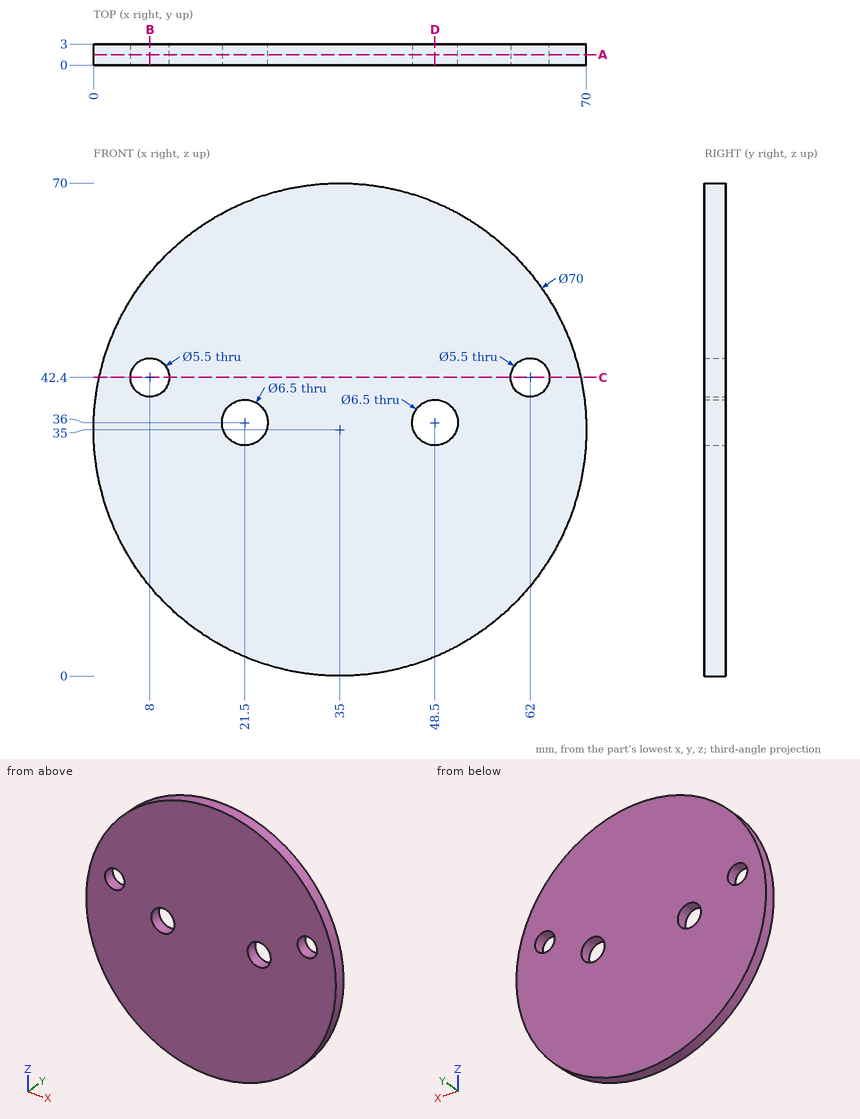
Here's the drawing with two shaded views (mm, measured from the low corner). I have some questions. Give positions to 0.01 mm unless a question says otherwise; leave off trailing zeros. Loops run counter-clockwise (first coordinate to the right, second up) from the corner with the lowest first, then second, coordinate; pieces in that order, holes last. Notation, with made-up numbers: (-24, 58.5) - (13, 58.5) arc R28 cw to (13, 83.5) - close; hole circle Ø7 at (52, 26.5). An arc over 180 degrees is marked (long way). Return JSON: item names as keys, results as strings.
1. I want a section at C-C on z = 42.4. Please give me the cut outline in (x, y).
Output values:
{"outline": "(0.79, 0) - (5.25, 0) - (5.25, 3) - (0.79, 3) - close; (10.75, 0) - (59.25, 0) - (59.25, 3) - (10.75, 3) - close; (64.75, 0) - (69.21, 0) - (69.21, 3) - (64.75, 3) - close"}
2. I want a section at B-B on x = 8. Please give me the cut outline in (y, z), and give its area (3 significant figures).
Output values:
{"outline": "(0, 12.73) - (3, 12.73) - (3, 39.65) - (0, 39.65) - close; (0, 45.15) - (3, 45.15) - (3, 57.27) - (0, 57.27) - close", "area": "117 mm²"}
3. If I drill on line 1 (X direction, y = 2.2, z = 39); line 2 (Z direction, x = 23.5, y = 0.3); line 3 (Z direction, x = 19, y = 0.85), over which ranges is the centre line in solid material (lowest first)?
Output values:
{"line 1": "x = 0.23 to 20.25, 22.75 to 47.25, 49.75 to 69.77", "line 2": "z = 1.94 to 33.44, 38.56 to 68.06", "line 3": "z = 3.87 to 33.92, 38.08 to 66.13"}
4. I want a section at D-D on x = 48.5. Please give me the cut outline in (y, z).
Output values:
{"outline": "(0, 2.71) - (3, 2.71) - (3, 32.75) - (0, 32.75) - close; (0, 39.25) - (3, 39.25) - (3, 67.29) - (0, 67.29) - close"}
5. I want a section at A-A on y = 1.5. Please give me the cut outline in (x, z), and give its area (3 significant figures).
Output values:
{"outline": "circle Ø70 at (35, 35); hole circle Ø5.5 at (8, 42.4); hole circle Ø6.5 at (21.5, 36); hole circle Ø6.5 at (48.5, 36); hole circle Ø5.5 at (62, 42.4)", "area": "3,730 mm²"}
6. I'm going to push flat-ended pins straight in: pin 1 Ø1.5 at (y, z) = (1, 31) entering from -X; pin 2 Ø9 at (x, z) = (62, 42.4) entering from -Y; pin 3 Ø5 at (x, z) = (21.5, 36) entering from -Y; pin 4 Ø1.5 at (y, z) = (1, 30) entering from +X. Where does each tip first touch, or does it pass through?
Output values:
{"pin 1": "stops at x = 0.15", "pin 2": "stops at y = 0", "pin 3": "passes through", "pin 4": "stops at x = 69.74"}
